Autodesk Inventor part; units mm, degrees
ref_plane "YZ Plane" through (0, 0, 0) normal (1, 0, 0) x (0, 1, 0)
ref_plane "XZ Plane" through (0, 0, 0) normal (0, 1, 0) x (-1, 0, 0)
ref_plane "XY Plane" through (0, 0, 0) normal (0, 0, 1) x (1, 0, 0)
sketch "Sketch1" plane through (0, 0, 0) normal (0, 1, 0) x (-1, 0, 0)
  line L0 (-75, 30) -> (75, 30)
  line L1 (75, 30) -> (75, -30)
  line L2 (75, -30) -> (-75, -30)
  line L3 (-75, -30) -> (-75, 30)
  line L4 (-75, 30) -> (75, -30) construction
  line L5 (75, 30) -> (-75, -30) construction
  line L6 (-80, 0) -> (-40, 0) construction
  line L7 (-80, -8.5) -> (-40, -8.5)
  line L8 (-40, 8.5) -> (-80, 8.5)
  arc A0 (-80, 8.5) -> (-80, -8.5) centre (-80, 0) ccw
  arc A1 (-40, -8.5) -> (-40, 8.5) centre (-40, 0) ccw
  circle A2 centre (55, 15) radius 3.25
  circle A3 centre (55, -15) radius 3.25
  circle A4 centre (35, 15) radius 3.25
  circle A5 centre (35, -15) radius 3.25
  point P0 (0, 0)
  point P1 (-60, 0)
  dimension "d0" = 60
  dimension "d1" = 150
  dimension "d2" = 60
  dimension "d3" = 40
  dimension "d4" = 17
  dimension "d5" = 6.5
  dimension "d6" = 15
  dimension "d7" = 30
  dimension "d8" = 20
  dimension "d9" = 20
extrude "Plate1" add sketch "Sketch1" along normal mid plane 10 contours L0 L1 L2 L3 L7 A1 L8 | L8 A1 L7 L3
extrude "Cut1" cut sketch "Sketch1" against normal mid plane 10 contours L8 A1 L7 L3 | L3 L7 A0 L8
sketch "Sketch2" plane through (0, -5, 0) normal (0, -1, 0) x (1, 0, 0)
  line L0 (-3, 12) -> (3, 12)
  line L1 (3, 12) -> (3, -12)
  line L2 (3, -12) -> (-3, -12)
  line L3 (-3, -12) -> (-3, 12)
  line L4 (75, 30) -> (-75, 30)
  point P0 (0, 0)
  point P1 (0, 12)
  dimension "d13" = 24
  dimension "d14" = 18
  dimension "d15" = 6
extrude "Cut2" cut sketch "Sketch2" against normal blind 10
fillet "Corner Round1" radius 6 4 edges at (75, 0, 30) (75, 0, 8.5) (75, 0, -8.5) (75, 0, -30)
equation "\"d11\" = Thickness"
equation "\"d16\" = Thickness"
equation "\"d10\" = Thickness"
equation "\"BendReliefDepth\" = 0.5 * Thickness"
properties part number "HCMUTE-CDT23-BAT_TRUC_CANG_TAI" material "Stainless Steel"
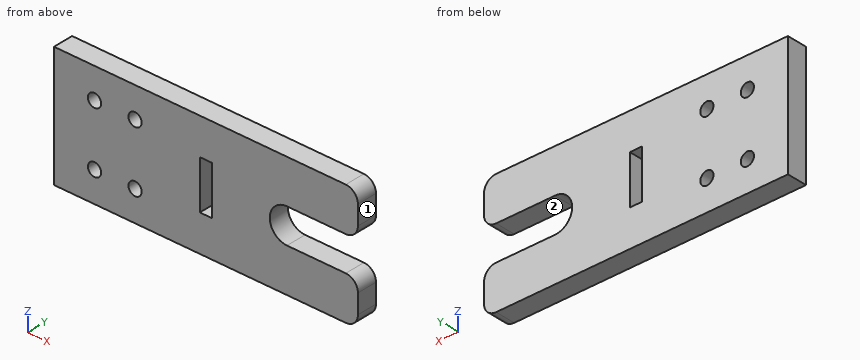
Here's how the part is built. I have some questions about the finished solid (model axes, mm). Face numbers are marked on the shaded views. A direction names the side the tool comes from. Coordinates: 2 decimals unless noted, no trailing zeros. Order: outer loops, then holes, each group sorted by start corner. A loop starts at its lowest first (then second) coordinate and runs counter-clockwise, first axis right, second up. Notation, with made-up numbers: M -4.5,13 L 25.5,13 A14 ccw 25.5,31 Z; hole C 31,-16 d2. An arc over 180 degrees is marked long. Answer as CSV lines item,"result". Start each with the question number.
1. For pin 1 (4 mm diameter, centred on y = 3, z = -3, fed in from +X); pin 2 (3 mm diameter, centred on y = 0, z = 10.5, fed in from +X); pin 3 (6 mm diameter, centred on x = -35, z = 15, fed in from -Y), each with a flat end and sliding along its axis, tell me the tip position at first contact or that it passes through.
2. I want a section at A-A, the plane x = 47. Write out the boundary of the cut face in (y, z), and give its area (3 significant figures).
3. I want a section at C-C, the plane x = -35. Write out the boundary of the cut face in (y, z).
4. On a 3-axis mill with a long thin cutter (end or side, diameter ignored), from which of +Z, -Z, +X, -X, +Y, -Y can I reach the whole of each face in a straight line? I mean the marked faces 1 and 2. Say none if no direction works.
5. I want a section at B-B, the plane y = -1.75. Write out the boundary of the cut face in (x, z), and give its area (3 significant figures).
6. I want a section at D-D, the plane z = -1.5. Write out the boundary of the cut face in (x, y).
7. I need wall thicknesses on line 1 (Z direction, x = -55, y = 3); line 2 (X direction, y = 0.25, z = -13); line 3 (X direction, y = 3.5, z = -16). Which ranges of each line are inside material? Lowest first, please. Write a range as [from, to].
Recorded:
1,pin 1,"stops at x = 33.13"
1,pin 2,"stops at x = 74.45"
1,pin 3,"passes through"
2,outline,"M -5,-30 L 5,-30 L 5,-8.5 L -5,-8.5 Z; M -5,8.5 L 5,8.5 L 5,30 L -5,30 Z"
2,area,"430 mm2"
3,outline,"M -5,-30 L 5,-30 L 5,-18.25 L -5,-18.25 Z; M -5,-11.75 L 5,-11.75 L 5,11.75 L -5,11.75 Z; M -5,18.25 L 5,18.25 L 5,30 L -5,30 Z"
4,face 1,"+Z, -Z, +X, +Y, -Y"
4,face 2,"+X, +Y, -Y"
5,outline,"M -75,-30 L 69,-30 A6 ccw 75,-24 L 75,-14.5 A6 ccw 69,-8.5 L 40,-8.5 A8.5 cw 40,8.5 L 69,8.5 A6 ccw 75,14.5 L 75,24 A6 ccw 69,30 L -75,30 Z; hole C -55,-15 d6.5; hole C -55,15 d6.5; hole C -35,-15 d6.5; hole C -35,15 d6.5; hole M -3,-12 L 3,-12 L 3,12 L -3,12 Z"
5,area,"7,980 mm2"
6,outline,"M -75,-5 L -3,-5 L -3,5 L -75,5 Z; M 3,-5 L 31.63,-5 L 31.63,5 L 3,5 Z"
7,line 1,"z = [-30, -18.25], [-11.75, 11.75], [18.25, 30]"
7,line 2,"x = [-75, -57.56], [-52.44, -37.56], [-32.44, 74.81]"
7,line 3,"x = [-75, -58.09], [-51.91, -38.09], [-31.91, 75]"
